Here's the drawing with two shaded views (mm, measured from the low corner). I have some questions. A direction names the side the tool comes from. Round coordinates to 2 decimals unless told otherwise and drop trailing zeros. Order: outer loops, then holes, each group sorted by start corner. A loop starts at its lowest first (then second) coordinate and runs counter-clockwise, first axis right, second up. Notation, with made-up numbers: (56.5, 25) -> (63.5, 25) arc R20 ccw to (63.5, 30) -> close; hole circle Ø8 at (-34.5, 63). An arc over 180 degrees is marked (long way). Use a Markdown table: item, result. Add a question column.
Q1. If we section it at D-D on x = 39: List the corners of the cut face in (y, z) for me, plus the area to 3 significant figures.
Q2. We'd pull the mould along X, two halves only. Please class the marked faces 1, 2, 3 and 4: +X half, -X half, draft (parallel to the pull), parting line (faces both ways), or undercut.
Q3. I'm going to push flat-ended pins straight in: pin 1 Ø6.5 at (y, z) = (30.5, 4.5) entering from +X (1 decimal); pin 2 Ø1 at (y, z) = (11, 43.5) entering from -X; pin 3 Ø6.5 at (y, z) = (21.5, 6) entering from -X (1 decimal); pin 4 Ø6.5 at (x, z) = (23.5, 5.5) entering from +Y. Where does each tip first touch, or does it pass through?
Q4. For the marked faces 5, 6 and 7, which set-ups out of +Z, -Z, +X, -X, +Y, -Y let a thin tool reach every point of the face, with its end or its side?
Q5. If we section it at C-C on y = 35: List the corners of the cut face in (x, z) for me (1 decimal).
Q6. I need wall thicknesses on line 1 along Z through (x, y) = (3, 27.5); line 2 along X through (y, z) = (19.5, 48) (1 decimal); line 3 along Z through (x, y) = (22, 18) (1 decimal). Which ranges of each line are inside material? Lowest first, please. Write a range as [from, to].
Q7. If we section it at B-B on x = 13.5: List the corners of the cut face in (y, z) for me, plus the area to 3 significant figures.
Q8. If we section it at A-A on z = 32: List the corners of the cut face in (x, y) for me, plus the area to 3 significant figures.
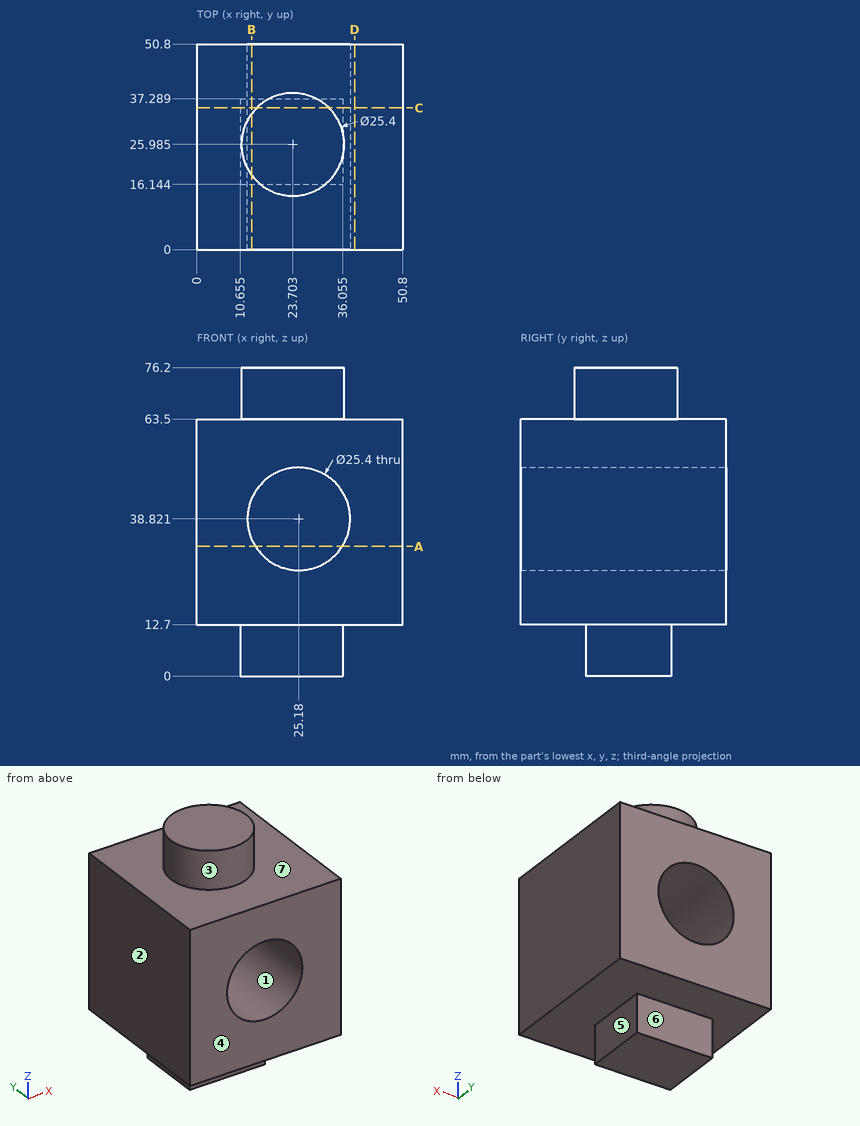
Answer below:
| question | item | result |
|---|---|---|
| 1 | outline | (0, 12.7) -> (50.8, 12.7) -> (50.8, 63.5) -> (0, 63.5) -> close |
| 1 | area | 2,580 mm² |
| 2 | face 1 | undercut |
| 2 | face 2 | -X half |
| 2 | face 3 | parting line |
| 2 | face 4 | draft |
| 3 | pin 1 | x = 36.1 |
| 3 | pin 2 | x = 0 |
| 3 | pin 3 | x = 10.7 |
| 3 | pin 4 | y = 37.29 |
| 4 | face 5 | -Z, +X, +Y, -Y |
| 4 | face 6 | -Z, +X, -X, +Y |
| 4 | face 7 | +Z |
| 5 | outline | (0, 12.7) -> (10.7, 12.7) -> (10.7, 0) -> (36.1, 0) -> (36.1, 12.7) -> (50.8, 12.7) -> (50.8, 63.5) -> (32.6, 63.5) -> (32.6, 76.2) -> (14.8, 76.2) -> (14.8, 63.5) -> (0, 63.5) -> close; hole circle Ø25.4 at (25.2, 38.8) |
| 6 | line 1 | [12.7, 63.5] |
| 6 | line 2 | [0, 16.4], [34, 50.8] |
| 6 | line 3 | [0, 26.5], [51.1, 76.2] |
| 7 | outline | (0, 12.7) -> (16.14, 12.7) -> (16.14, 0) -> (37.29, 0) -> (37.29, 12.7) -> (50.8, 12.7) -> (50.8, 33.83) -> (0, 33.83) -> close; (0, 43.81) -> (50.8, 43.81) -> (50.8, 63.5) -> (33.55, 63.5) -> (33.55, 76.2) -> (18.42, 76.2) -> (18.42, 63.5) -> (0, 63.5) -> close |
| 7 | area | 2,530 mm² |
| 8 | outline | (0, 0) -> (14.47, 0) -> (14.47, 50.8) -> (0, 50.8) -> close; (35.89, 0) -> (50.8, 0) -> (50.8, 50.8) -> (35.89, 50.8) -> close |
| 8 | area | 1,490 mm² |
